```python
from build123d import *

# Parameters (mm, degrees)
SKETCH_R    = 3
PAD_DEPTH   = 3.175
FILLET_R    = 3
FILLET001_R = 1


with BuildPart() as part:
    # Sketch → Pad (new body)
    with BuildSketch(Plane.XZ):
        with BuildLine():
            Line((0, 0), (20, 0))
            ThreePointArc((70, 50), (39.553951, 30.446049), (20, 0))
            Line((70, 50), (70, 70))
            Line((70, 70), (0, 70))
            Line((0, 70), (0, 0))
        make_face()
        with Locations((10, 40)):
            Circle(SKETCH_R, mode=Mode.SUBTRACT)
        with Locations((10, 8)):
            Circle(SKETCH_R, mode=Mode.SUBTRACT)
        with Locations((30, 60)):
            Circle(SKETCH_R, mode=Mode.SUBTRACT)
        with Locations((62, 60)):
            Circle(SKETCH_R, mode=Mode.SUBTRACT)
        with BuildLine():
            Line((47.893188, 50), (20, 50))
            Line((20, 50), (20, 22.106812))
            ThreePointArc((47.893188, 50), (32.482884, 37.517116), (20, 22.106812))
        make_face(mode=Mode.SUBTRACT)
    extrude(amount=PAD_DEPTH)

    # Fillet
    fillet_edges = [part.edges().sort_by_distance(p)[0] for p in [
        (20, -1.5875, 22.106812),
        (47.893188, -1.5875, 50),
        (20, -1.5875, 50),
    ]]
    fillet(fillet_edges, radius=FILLET_R)

    # Fillet001
    fillet001_edges = [part.edges().sort_by_distance(p)[0] for p in [
        (70, -1.5875, 50),
        (70, -1.5875, 70),
        (20, -1.5875, 0),
        (0, -1.5875, 0),
        (0, -1.5875, 70),
    ]]
    fillet(fillet001_edges, radius=FILLET001_R)


solid = part.part
```
Verification items for the finished model (mm, model axes). A direction names the side the tool comes from. Round coordinates to 2 decimals unless told otherwise and drop trailing zeros. Write each loop counter-clockwise with the first axis right and the second up, starting at its lowest first coordinate (ties: lowest second). Pieces come first, ordered by that corner, then holes.
1. Section check A-A on x = 10. Enter the section's corners in (y, z) (3 decimals).
2. Draft check along X on faces 3 (the cylindrical face through (32.589, -1.565, 37.623)), 4 (the flat face through (35, -2, 70)), 5 (the cylindrical face through (39.91, -1.57, 30.8)). Enter one of: +X half, -X half, draft (parallel to the pull), parting line (faces both ways), or undercut.
3. Section check D-D on x = 34.5. Enter the section's corners in (y, z) (3 decimals).
4. Scan lines: L1, parallel to Z at x = 10, y = -2.45; L2, parallel to Z at x = 30, y = -0.75; L3, parallel to Z at x = 19.5, y = -0.5. Record each from-to range of solid material in increasing order.
5. Section check B-B on y = -2.5. Enter the section's corners in (x, z).
6. Section check C-C on z = 60. Enter the section's corners in (x, y) (3 decimals).
7. Access from +Z, -Z, +X, -X, +Y, -Y to the whole of each face (thin tool, end or side, straight path). Record for faces 1 (the flat face through (70, -2, 60)), 2 (the flat face through (20, -2, 39)).
Answer:
1. outline: (-3.175, 0) - (0, 0) - (0, 5) - (-3.175, 5) - close; (-3.175, 11) - (0, 11) - (0, 37) - (-3.175, 37) - close; (-3.175, 43) - (0, 43) - (0, 70) - (-3.175, 70) - close
2. face 3: undercut
2. face 4: draft
2. face 5: +X half
3. outline: (-3.175, 24.926) - (0, 24.926) - (0, 39.475) - (-3.175, 39.475) - close; (-3.175, 50) - (0, 50) - (0, 70) - (-3.175, 70) - close
4. L1: z = 0 to 5, 11 to 37, 43 to 70
4. L2: z = 19.05 to 34.94, 50 to 57, 63 to 70
4. L3: z = 0.02 to 70
5. outline: (0, 1) arc R1 ccw to (1, 0) - (19.31, 0) arc R1 ccw to (20.24, 0.64) arc R85 cw to (69.36, 49.76) arc R1 ccw to (70, 50.69) - (70, 69) arc R1 ccw to (69, 70) - (1, 70) arc R1 ccw to (0, 69) - close; hole circle Ø6 at (10, 8); hole circle Ø6 at (10, 40); hole (20, 31.4) arc R3 ccw to (25.35, 29.53) arc R95 cw to (40.47, 44.65) arc R3 ccw to (38.6, 50) - (23, 50) arc R3 ccw to (20, 47) - close; hole circle Ø6 at (30, 60); hole circle Ø6 at (62, 60)
6. outline: (0, -3.175) - (27, -3.175) - (27, 0) - (0, 0) - close; (33, -3.175) - (59, -3.175) - (59, 0) - (33, 0) - close; (65, -3.175) - (70, -3.175) - (70, 0) - (65, 0) - close
7. face 1: +Z, -Z, +X, +Y, -Y
7. face 2: +Y, -Y
